Could you check a few things on this model? Use its own coordinates, in mm. Face numbers are marked on the shaded views. A direction names the side the tool comes from. Round coordinates to 2 decimals unless told otherwise and drop trailing zeros. Order: outer loops, then holes, each group sorted by start corner. A loop starts at its lowest first (then second) coordinate and runs counter-clockwise, first axis right, second up. Notation, with made-up numbers: M 16,33 L 62,33 A12 ccw 62,41 Z; hole C -9,12.5 d1. An arc over 180 degrees is marked long. Write each question's results on one line, items separated by ' | '. Start each with the question number.
1. We'd pull the mould along X, two halves only. Please class the marked faces 4, 5 and 6: released by +X, released by -X, zero draft, split by the parting line, or undercut.
2. Suppose I cut it at C-C on x = -1. Write out the boundary of the cut face in (y, z), and give its area (3 significant figures).
3. Suppose I cut it at B-B on x = 2.5. Write out the boundary of the cut face in (y, z).
4. I'm going to push flat-ended pins straight in: pin 1 (1.5 mm diameter, centred on x = 15.5, z = 2, fed in from -Y); pin 2 (1 mm diameter, centred on y = 1.5, z = 2, fed in from -X); pin 3 (1.1 mm diameter, centred on x = -15, z = 1, fed in from -Y). Where does each tip first touch, or does it pass through?
5. Please list where these lines run through material, in increasing order: L1, parallel to Y at x = -15.5, z = 1.25; L2, parallel to X at y = 2.5, z = 1.5; L3, parallel to Y at x = 0, z = 2.75 (3 decimals).
6. For the marked faces 1, 2 and 3, which set-ups out of +Z, -Z, +X, -X, +Y, -Y let a thin tool reach every point of the face, with its end or its side?
7. Suppose I cut it at A-A on y = 0. Write out the boundary of the cut face in (x, z).
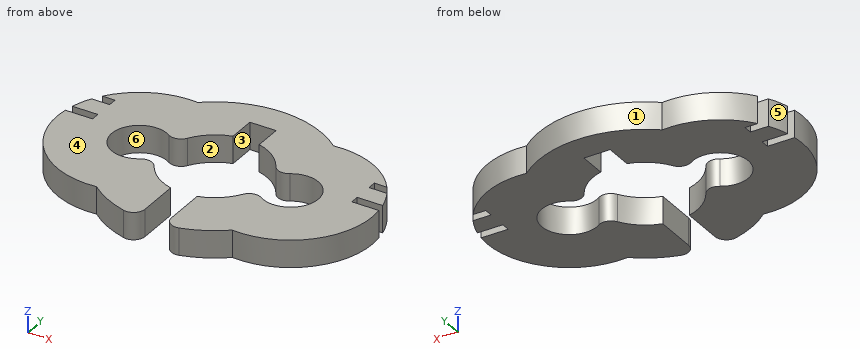
from build123d import *

# Parameters (mm, degrees)
EXTRUDE_1_DEPTH     = 3
SKETCH_2_W          = 3
SKETCH_2_H          = 0.95
CUT_EXTRUDE_1_DEPTH = 3
FILLET_1_R          = 1.27


with BuildPart() as part:
    # 스케치1 → 보스-돌출1 (new body)
    with BuildSketch(Plane.XY):
        with BuildLine():
            Line((-1.4475, 8.528649813), (1.4475, 8.528649813))
            Line((1.4475, 8.528649813), (1.4475, 5.528649813))
            ThreePointArc((1.4475, 5.528649813), (4.105207543, 3.975989943), (5.572102386, 1.27))
            ThreePointArc((5.572102386, 1.27), (11.390915263, 0), (5.572102386, -1.27))
            ThreePointArc((5.572102386, -1.27), (4.110599393, -3.970415297), (1.4625, -5.524700784))
            Line((1.4625, -5.524700784), (1.4625, -11.623352303))
            ThreePointArc((1.4625, -11.623352303), (4.663454339, -10.746786433), (7.490136969, -9.007722974))
            ThreePointArc((7.490136969, -9.007722974), (17.390915263, 0), (7.490136969, 9.007722974))
            ThreePointArc((7.490136969, 9.007722974), (0, 11.715), (-7.490136969, 9.007722974))
            ThreePointArc((-7.490136969, 9.007722974), (-17.390915263, 0), (-7.490136969, -9.007722974))
            ThreePointArc((-7.490136969, -9.007722974), (-4.663454339, -10.746786433), (-1.4625, -11.623352303))
            Line((-1.4625, -11.623352303), (-1.4625, -5.524700784))
            ThreePointArc((-1.4625, -5.524700784), (-4.110599393, -3.970415297), (-5.572102386, -1.27))
            ThreePointArc((-5.572102386, -1.27), (-11.390915263, 0), (-5.572102386, 1.27))
            ThreePointArc((-5.572102386, 1.27), (-4.105207543, 3.975989943), (-1.4475, 5.528649813))
            Line((-1.4475, 5.528649813), (-1.4475, 8.528649813))
        make_face()
    extrude(amount=EXTRUDE_1_DEPTH)

    # 스케치2 → 컷-돌출1 (cut)
    with BuildSketch(Plane.XY.offset(3)):
        with Locations((15.801341687, 1.745)):
            Rectangle(SKETCH_2_W, SKETCH_2_H)
        with Locations((-15.801341687, 4.795)):
            Rectangle(SKETCH_2_W, SKETCH_2_H)
        with Locations((-15.801341687, 1.745)):
            Rectangle(SKETCH_2_W, SKETCH_2_H)
        with Locations((15.801341687, 4.795)):
            Rectangle(SKETCH_2_W, SKETCH_2_H)
    extrude(amount=-CUT_EXTRUDE_1_DEPTH, mode=Mode.SUBTRACT)

    # 필렛1
    fillet_1_edges = [part.edges().sort_by_distance(p)[0] for p in [
        (-5.572102386, 1.27, 1.5),
        (-5.572102386, -1.27, 1.5),
        (-1.4625, -11.623352303, 1.5),
        (1.4625, -11.623352303, 1.5),
        (5.572102386, -1.27, 1.5),
        (5.572102386, 1.27, 1.5),
    ]]
    fillet(fillet_1_edges, radius=FILLET_1_R)


solid = part.part
Filled sheet:
1) face 4: zero draft | face 5: released by -X | face 6: undercut
2) outline: M 8.53,0 L 11.67,0 L 11.67,3 L 8.53,3 Z | area: 9.43 mm^2
3) outline: M -11.33,0 L -5.14,0 L -5.14,3 L -11.33,3 Z; M 5.14,0 L 11.45,0 L 11.45,3 L 5.14,3 Z
4) pin 1: stops at y = -6.39 | pin 2: stops at x = -17.34 | pin 3: stops at y = -6.68
5) L1: y = -5.54 to 1.27, 2.22 to 4.32, 5.27 to 5.54 | L2: x = -17.04 to -10.09, -6.59 to -5.37, 5.37 to 6.59, 10.09 to 17.04 | L3: y = 8.529 to 11.715
6) face 1: +Z, -Z, +Y | face 2: +Z, -Z | face 3: +Z, -Z, -Y
7) outline: M -17.39,0 L -11.39,0 L -11.39,3 L -17.39,3 Z; M 11.39,0 L 17.39,0 L 17.39,3 L 11.39,3 Z
